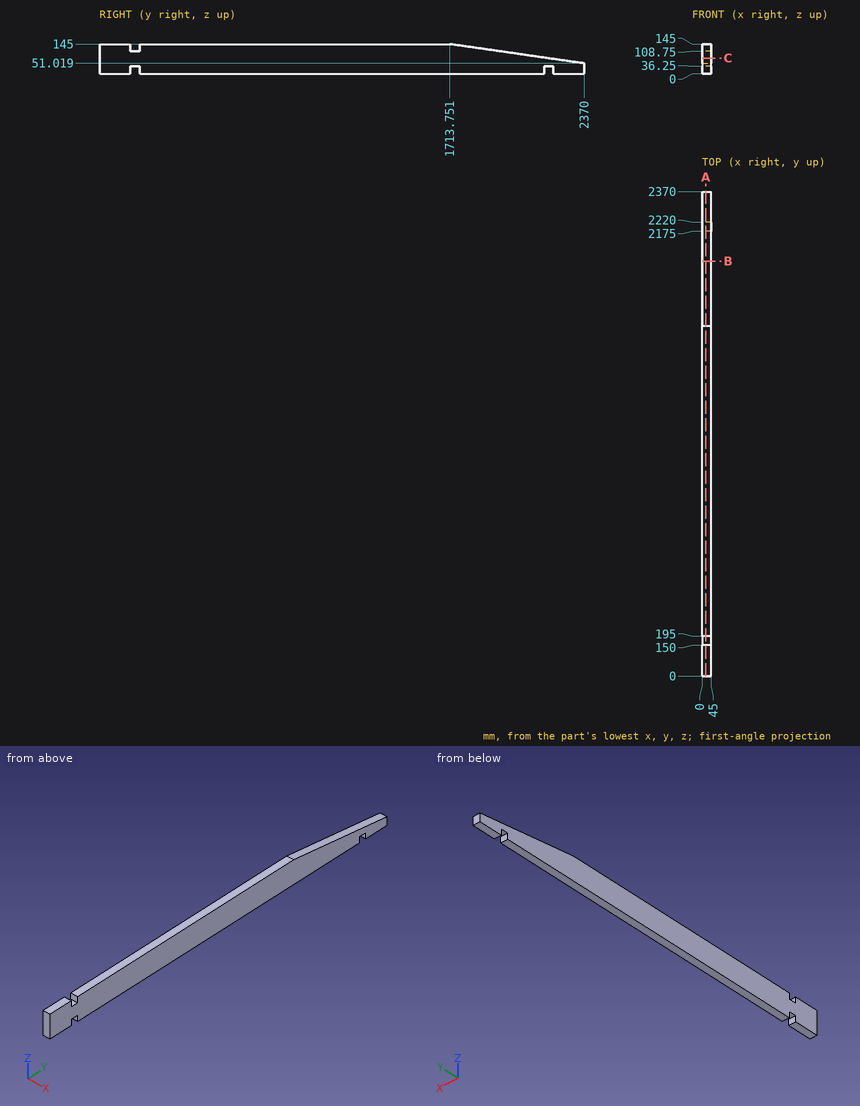
Source: three-view drawing plus pictorial views. Frame: mm from the lowest corner of the part. Coordinates: 2 decimals unless noted, no trailing zeros. Loops run counter-clockwise (first coordinate to the right, second up) from the corner with the lowest first, then second, coordinate; pieces in that order, holes last. Notation, with made-up numbers: (40, 58) -> (69, 58) arc R17 cw to (69, 73) -> close; hole circle Ø7 at (56.5, -34). An arc over 180 degrees is marked (long way). Answer in a Markdown table with one row per item. Add a question column.
Q1. Ray query, line 1 along Y through (x, z) = (43, 20); line 2 along Z through (x, y) = (23, 1750.5); line 3 along Z through (x, y) = (2, 1925). Return the intervals inside material, ascending.
Q2. Section C-C on z = 76. Return the cut outline in (x, y).
Q3. Section A-A on x = 19. Return the cut outline in (y, z), and give its area (3 significant figures).
Q4. Section B-B on y = 2029.5. Return the cut outline in (x, z), and give its area (3 significant figures).
Q5. Contact query for flat-ended pins moving along their axis: pin 1 Ø6 at (y, z) = (1551, 56) entering from -X; pin 2 Ø22.5 at (x, y) = (15, 176) entering from +Z; pin 3 Ø22.5 at (x, y) = (23.5, 170.5) entering from -Z. Output: stop coordinate, or through.
Computed values:
| question | item | result |
|---|---|---|
| 1 | line 1 | y = 0 to 150, 195 to 2175, 2220 to 2370 |
| 1 | line 2 | z = 0 to 139.74 |
| 1 | line 3 | z = 0 to 114.75 |
| 2 | outline | (0, 0) -> (45, 0) -> (45, 2195.56) -> (0, 2195.56) -> close |
| 3 | outline | (0, 0) -> (150, 0) -> (150, 36.25) -> (195, 36.25) -> (195, 0) -> (2175, 0) -> (2175, 36.25) -> (2220, 36.25) -> (2220, 0) -> (2370, 0) -> (2370, 51.02) -> (1713.75, 145) -> (195, 145) -> (195, 108.75) -> (150, 108.75) -> (150, 145) -> (0, 145) -> close |
| 3 | area | 308,000 mm^2 |
| 4 | outline | (0, 0) -> (45, 0) -> (45, 99.78) -> (0, 99.78) -> close |
| 4 | area | 4,490 mm^2 |
| 5 | pin 1 | stops at x = 0 |
| 5 | pin 2 | stops at z = 108.75 |
| 5 | pin 3 | stops at z = 36.25 |
